The listing builds one solid part. Answer for the finished solid, in the listing's coordinates (mm). Coordinates: 2 decimals unless noted, no trailing zeros. Order: outer loops, then holes, each group sorted by start corner. A loop starts at its lowest first (then second) coordinate and runs counter-clockwise, first axis right, second up.
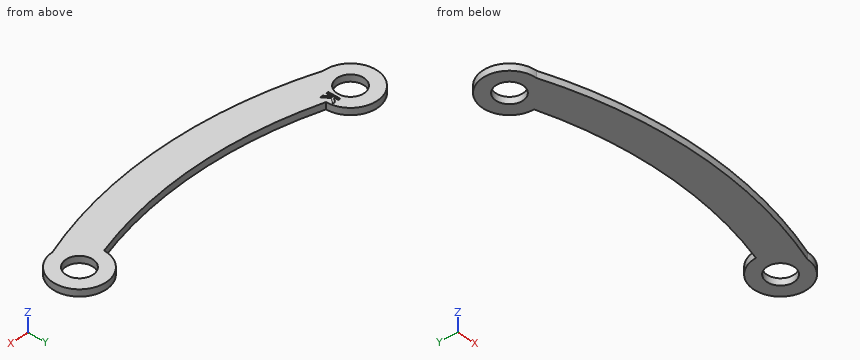
from build123d import *

# Parameters (mm, degrees)
ESQUISSE1_R             = 3.985
BOSS_EXTRU_1_DEPTH      = 2
ENL_V_MAT_EXTRU_1_DEPTH = 0.3


with BuildPart() as part:
    # Esquisse1 → Boss.-Extru.1 (new body)
    with BuildSketch(Plane(origin=(0, 0, 0), x_dir=(0, 1, 0), z_dir=(0, 0, 1))):
        with BuildLine():
            ThreePointArc((-7.89, 0), (5.579072504, -5.579072504), (0, 7.89))
            ThreePointArc((0, 7.89), (-5.478052173, 43.5), (0, 79.11))
            ThreePointArc((0, 79.11), (5.579072504, 92.579072504), (-7.89, 87))
            ThreePointArc((-7.89, 87), (-15.478052173, 43.5), (-7.89, 0))
        make_face()
        with Locations(Location((0, 0, 0), (0, 0, 270))):
            Circle(ESQUISSE1_R, mode=Mode.SUBTRACT)
        with Locations(Location((0, 87, 0), (0, 0, 270))):
            Circle(ESQUISSE1_R, mode=Mode.SUBTRACT)
    extrude(amount=BOSS_EXTRU_1_DEPTH)

    # Esquisse2 → Enlèv. mat.-Extru.1 (cut)
    with BuildSketch(Plane.XY.offset(2)):
        Polygon((-82.098700293, 1.451884906), (-81.470495165, 1.451884906), (-81.470495165, 0.220013912), (-80.477706704, 1.451884906), (-79.684737954, 1.451884906), (-80.932033627, -0.096192018), (-79.563443883, -2.048115094), (-80.3199543, -2.048115094), (-81.470495165, -0.406788973), (-81.470495165, -2.048115094), (-82.098700293, -2.048115094), align=None)
    extrude(amount=-ENL_V_MAT_EXTRU_1_DEPTH, mode=Mode.SUBTRACT)


solid = part.part
(1) Find section D-D on x = -68.5. Determine the outline of the cut face in (y, z).
(2) Find the intervals of material crossed by probe 1 along Y at (x, z) = (-87, 0.4) (3 decimals); probe 2 along Y at (x, z) = (-85, 1.1); probe 3 along X at (y, z) = (6.5, 1.45), in increasing order.
(3) Given pin 1 Ø0.8 at (x, y) = (-80.5, -1) entering from +Z; pin 2 Ø7 at (x, y) = (0, 0) entering from +Z, each flat-ended and moving along its own axis, determine where each tip first touches the part or whether it passes through.
(4) Find section B-B on x = -2. Determine the outline of the cut face in (y, z).
(5) Find section C-C on x = -23.5. Determine the outline of the cut face in (y, z).
(6) Find section A-A on z = 1.4. Determine the outline of the cut face in (x, y) (3 decimals).
Resolved:
1. outline: (-13.02, 0) - (-2.81, 0) - (-2.81, 2) - (-13.02, 2) - close
2. probe 1: y = -7.89 to -3.985, 3.985 to 7.89
2. probe 2: y = -8.59 to -3.45, 3.45 to 7.63
2. probe 3: x = -91.47 to -82.53, -4.47 to 4.47
3. pin 1: stops at z = 2
3. pin 2: passes through
4. outline: (-8.59, 0) - (-3.45, 0) - (-3.45, 2) - (-8.59, 2) - close; (3.45, 0) - (7.63, 0) - (7.63, 2) - (3.45, 2) - close
5. outline: (-13.91, 0) - (-3.78, 0) - (-3.78, 2) - (-13.91, 2) - close
6. outline: (-87, -7.89) arc R128.48 ccw to (0, -7.89) arc R7.89 ccw (long way) to (-7.89, 0) arc R118.48 cw to (-79.11, 0) arc R7.89 ccw (long way) to start; hole circle Ø7.97 at (-87, 0); hole circle Ø7.97 at (0, 0)
